```python
from build123d import *

# Parameters (mm, degrees)
ESQUISSE1_W             = 49
ESQUISSE1_H             = 29
ESQUISSE1_W_2           = 41
ESQUISSE1_H_2           = 21
BOSS_EXTRU_1_DEPTH      = 19
CONG_1_R                = 3
CONG_2_R                = 2
ESQUISSE2_W             = 15
ESQUISSE2_H             = 10.5
BOSS_EXTRU_2_DEPTH      = 19
ESQUISSE3_W             = 15
ESQUISSE3_H             = 10.5
BOSS_EXTRU_3_DEPTH      = 19
ENL_V_MAT_EXTRU_1_REACH = 83.444
ESQUISSE5_R             = 3
ENL_V_MAT_EXTRU_2_REACH = 83.444
ENL_V_MAT_EXTRU_3_REACH = 73.505
ESQUISSE8_R             = 3
ENL_V_MAT_EXTRU_4_REACH = 73.505


with BuildPart() as part:
    # Esquisse1 → Boss.-Extru.1 (new body)
    with BuildSketch(Plane(origin=(0, 0, 0), x_dir=(1, 0, 0), z_dir=(0, 1, 0))):
        with Locations((-32.579514124, -18.656539988)):
            Rectangle(ESQUISSE1_W, ESQUISSE1_H)
        with Locations((-32.579514124, -18.656539988)):
            Rectangle(ESQUISSE1_W_2, ESQUISSE1_H_2, mode=Mode.SUBTRACT)
    extrude(amount=BOSS_EXTRU_1_DEPTH)

    # Congé1
    cong_1_edges = [part.edges().sort_by_distance(p)[0] for p in [
        (-57.079514124, 9.5, 4.156539988),
        (-8.079514124, 9.5, 4.156539988),
        (-8.079514124, 9.5, 33.156539988),
        (-57.079514124, 9.5, 33.156539988),
    ]]
    fillet(cong_1_edges, radius=CONG_1_R)

    # Congé2
    cong_2_edges = [part.edges().sort_by_distance(p)[0] for p in [
        (-53.079514124, 9.5, 8.156539988),
        (-53.079514124, 9.5, 29.156539988),
        (-12.079514124, 9.5, 29.156539988),
        (-12.079514124, 9.5, 8.156539988),
    ]]
    fillet(cong_2_edges, radius=CONG_2_R)

    # Esquisse2 → Boss.-Extru.2 (add)
    with BuildSketch(Plane(origin=(-8.079514124, 0, 0), x_dir=(0, 0, -1), z_dir=(1, 0, 0))):
        with Locations((-18.656539988, 5.5)):
            Rectangle(ESQUISSE2_W, ESQUISSE2_H)
    extrude(amount=BOSS_EXTRU_2_DEPTH)

    # Esquisse3 → Boss.-Extru.3 (add)
    with BuildSketch(Plane.ZY.offset(57.079514124)):
        with Locations((18.656539988, 5.5)):
            Rectangle(ESQUISSE3_W, ESQUISSE3_H)
    extrude(amount=BOSS_EXTRU_3_DEPTH)

    # Esquisse5 → Enlèv. mat.-Extru.1 (cut, up to next)
    with BuildSketch(Plane(origin=(0, 0, 11.156539988), x_dir=(-1, 0, 0), z_dir=(0, 0, -1)), mode=Mode.PRIVATE) as enl_v_mat_extru_1_sk1:
        with Locations(Location((60.079514124, 5.5, 0), (0, 0, 180))):
            Circle(ESQUISSE5_R)
    enl_v_mat_extru_1_tool1 = extrude(enl_v_mat_extru_1_sk1.sketch, amount=-ENL_V_MAT_EXTRU_1_REACH, mode=Mode.PRIVATE) & part.part
    add(enl_v_mat_extru_1_tool1.solids().sort_by_distance((-60.079514, 5.5, 11.15654))[0], mode=Mode.SUBTRACT)

    # Esquisse7 → Enlèv. mat.-Extru.2 (cut, up to next)
    with BuildSketch(Plane(origin=(0, 0, 11.156539988), x_dir=(-1, 0, 0), z_dir=(0, 0, -1)), mode=Mode.PRIVATE) as enl_v_mat_extru_2_sk1:
        with BuildLine():
            Line((60.079514124, 0.25), (76.079514124, 0.25))
            Line((76.079514124, 0.25), (76.079514124, 10.75))
            Line((76.079514124, 10.75), (60.079514124, 10.75))
            ThreePointArc((60.079514124, 10.75), (65.329514124, 5.5), (60.079514124, 0.25))
        make_face()
    enl_v_mat_extru_2_tool1 = extrude(enl_v_mat_extru_2_sk1.sketch, amount=-ENL_V_MAT_EXTRU_2_REACH, mode=Mode.PRIVATE) & part.part
    add(enl_v_mat_extru_2_tool1.solids().sort_by_distance((-70.083379, 5.5, 11.15654))[0], mode=Mode.SUBTRACT)

    # Esquisse8 → Enlèv. mat.-Extru.3 (cut, up to next)
    with BuildSketch(Plane(origin=(0, 0, 11.156539988), x_dir=(-1, 0, 0), z_dir=(0, 0, -1)), mode=Mode.PRIVATE) as enl_v_mat_extru_3_sk1:
        with Locations((5.079514124, 5.5)):
            Circle(ESQUISSE8_R)
    enl_v_mat_extru_3_tool1 = extrude(enl_v_mat_extru_3_sk1.sketch, amount=-ENL_V_MAT_EXTRU_3_REACH, mode=Mode.PRIVATE) & part.part
    add(enl_v_mat_extru_3_tool1.solids().sort_by_distance((-5.079514, 5.5, 11.15654))[0], mode=Mode.SUBTRACT)

    # Esquisse9 → Enlèv. mat.-Extru.4 (cut, up to next)
    with BuildSketch(Plane(origin=(0, 0, 11.156539988), x_dir=(-1, 0, 0), z_dir=(0, 0, -1)), mode=Mode.PRIVATE) as enl_v_mat_extru_4_sk1:
        with BuildLine():
            Line((5.079514124, 0.25), (-10.920485876, 0.25))
            Line((-10.920485876, 0.25), (-10.920485876, 10.75))
            Line((-10.920485876, 10.75), (5.079514124, 10.75))
            ThreePointArc((5.079514124, 10.75), (-0.170485876, 5.5), (5.079514124, 0.25))
        make_face()
    enl_v_mat_extru_4_tool1 = extrude(enl_v_mat_extru_4_sk1.sketch, amount=-ENL_V_MAT_EXTRU_4_REACH, mode=Mode.PRIVATE) & part.part
    add(enl_v_mat_extru_4_tool1.solids().sort_by_distance((4.924351, 5.5, 11.15654))[0], mode=Mode.SUBTRACT)


solid = part.part
```
Read the model definition and answer for the solid it produces. Units are mm, in the model's axes. A direction names the side the tool comes from. Give positions to 0.01 mm unless a question says otherwise; leave off trailing zeros. Write each loop counter-clockwise with the first axis right and the second up, starting at its lowest first coordinate (ties: lowest second). Pieces come first, ordered by that corner, then holes. Notation, with made-up numbers: (78, -25) -> (134, -25) arc R33 ccw to (134, 6) -> close; hole circle Ø8 at (8, 28.5). An arc over 180 degrees is marked (long way). Answer in a Markdown table with one row per item.
1) Straight lines are drawn through the part: line 1 (Z direction, x = -27, y = 5.25); line 2 (X direction, y = 2.75, z = 27.25); line 3 (X direction, y = 6, z = 22.5). For each, find the intervals that lie inside material, in ascending order. Write a range as [from, to].
Results list:
| item | result |
|---|---|
| line 1 | [4.16, 8.16], [29.16, 33.16] |
| line 2 | [-57.08, -53.08], [-12.08, -8.08] |
| line 3 | [-65.31, -63.04], [-57.12, -53.08], [-12.08, -8.04], [-2.12, 0.15] |
2) Each of these flat-tipped pins is pushed along its axis until it touches: pin 1 Ø4 at (y, z) = (16, 28.5) entering from +X; pin 2 Ø8 at (y, z) = (8, 9.5) entering from +X; pin 3 Ø6.5 at (x, y) = (-3, 4) entering from +Z; pin 4 Ø0.9 at (x, z) = (-6, 18) entering from +Y. Where does it stop, or does it pass through?
Results list:
| item | result |
|---|---|
| pin 1 | x = -8.08 |
| pin 2 | x = 0.17 |
| pin 3 | z = 26.16 |
| pin 4 | y = 10.75 |
3) Section A-A on z = 13.25 is taken. Give the vertices of the cut face in (x, y), plus the area to 3 significant figures.
Results list:
| item | result |
|---|---|
| outline | (-60.08, 0.25) -> (-57.08, 0.25) -> (-57.08, 0) -> (-53.08, 0) -> (-53.08, 19) -> (-57.08, 19) -> (-57.08, 10.75) -> (-60.08, 10.75) arc R5.25 ccw to start; (-12.08, 0) -> (-8.08, 0) -> (-8.08, 0.25) -> (-5.08, 0.25) arc R5.25 ccw to (-5.08, 10.75) -> (-8.08, 10.75) -> (-8.08, 19) -> (-12.08, 19) -> close; hole circle Ø6 at (-60.08, 5.5); hole circle Ø6 at (-5.08, 5.5) |
| area | 245 mm^2 |
4) A tool of negligible diameter and unlimited length cuts with its end or side. For faces 1 (the flat face through (-2, 7, 11.157)), 2 (the flat face through (-63, 7, 26.157)), 3 (the cylindrical face through (-52.478, 9.633, 28.586)), 4 (the flat face through (-7, 0.25, 19)), from which of +Z, -Z, +X, -X, +Y, -Y can it reach the whole face along a straight path? Write none if from no direction.
Results list:
| item | result |
|---|---|
| face 1 | -Z, +X, +Y, -Y |
| face 2 | +Z, -X, +Y, -Y |
| face 3 | +Y, -Y |
| face 4 | +Z, -Z, +X, -Y |
5) Determine the mould class of faces 5 (the cylindrical face through (-56.224, 9.633, 5.059)), 6 (the cylindrical face through (-52.48, 9.63, 8.73)), 7 (the cylindrical face through (-56.224, 9.633, 32.254)) for opening direction Z: released by +Z, released by -Z, zero draft, split by the parting line, or undercut.
Results list:
| item | result |
|---|---|
| face 5 | released by -Z |
| face 6 | undercut |
| face 7 | released by +Z |
6) Section C-C on y = 4 is taken. Count the separate pieces of the cut face and the enclosed holes in it, plus the area to 3 significant figures.
Results list:
| item | result |
|---|---|
| separate pieces | 3 |
| enclosed holes | 1 |
| area | 641 mm^2 |
7) Section B-B on x = -43 is taken. Give the vertices of the cut face in (y, z).
Results list:
| item | result |
|---|---|
| outline | (0, 4.16) -> (19, 4.16) -> (19, 8.16) -> (0, 8.16) -> close; (0, 29.16) -> (19, 29.16) -> (19, 33.16) -> (0, 33.16) -> close |
